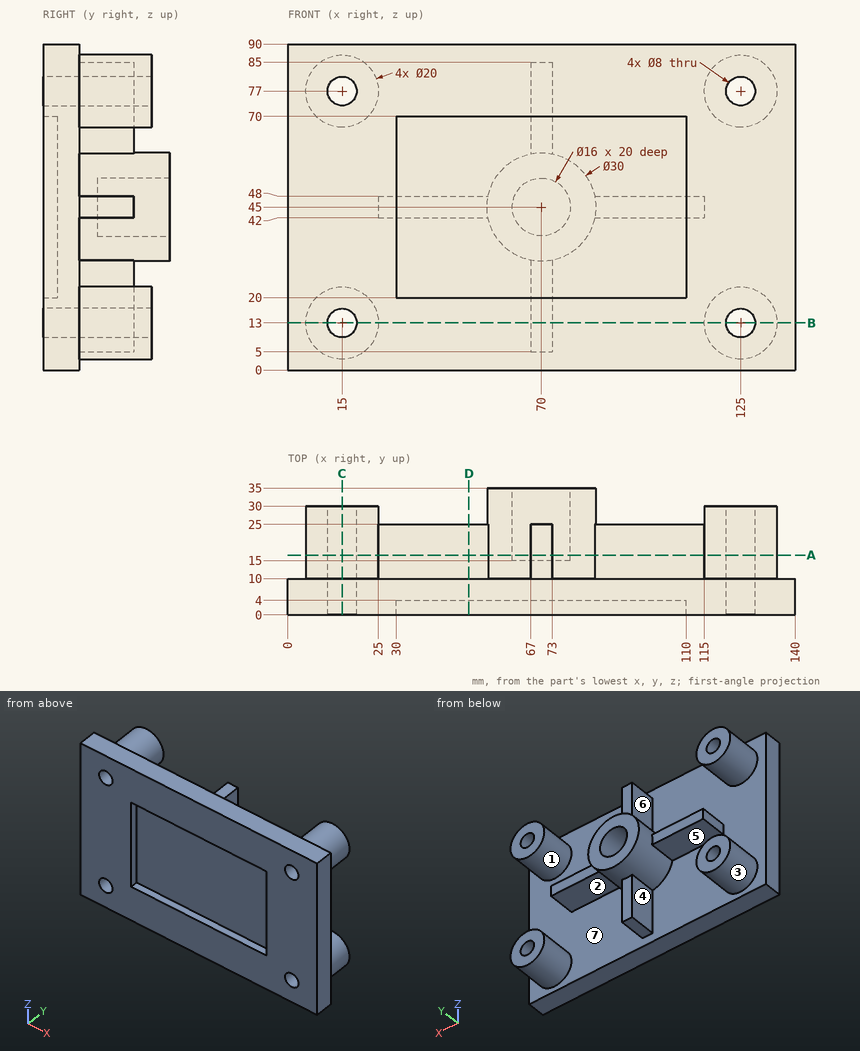
Input: dimensioned drawing with shaded views. Units: mm. Origin: part minimum x, y, z. A direction names the side the tool comes from. Give positions to 0.01 mm unless a question says otherwise; leave off trailing zeros. Write each loop counter-clockwise with the first axis right and the second up, starting at its lowest first coordinate (ties: lowest second). Pieces come first, ordered by that corner, then holes.
1. Reachability of the marked faces 5, 6 and 7 from +Z, -Z, +X, -X, +Y, -Y: full face, straight path, thin tool, end or side. Return the list, or none.
2. Pin query (flat end, axial travel): P1, Ø12, axis at x = 84, z = 33.5, coming from the -Y side; P2, Ø5, axis at y = 18, z = 10.5, coming from the +X side; P3, Ø6.5, axis at x = 40.5, z = 44.5, coming from the +Y side. Return the tip coordinate at first contact, or that it passes through.
3. Line query: probe 1 along X at (y, z) = (10.5, 77); probe 2 along X at (y, z) = (3.5, 31); probe 3 along Z at (x, y) = (17, 23.5). Output: solid intervals per line, ascending.
4. Section query A-A, the plane y = 16.5. Count the separate pieces of the cut face and the enclosed holes in it, then the cut area to 3 significant figures.
5. Section query B-B, the plane z = 13. Return loops of the section in (x, y), then the cut area to 3 significant figures.
6. Draft query along Z for the marked faces 1, 2, 3 and 4. Return one class per face: released by +Z, released by -Z, zero draft, split by the parting line, or undercut.
7. Section query D-D, the plane x = 50. Return loops of the section in (y, z), then the cut area to 3 significant figures.
8. Section query C-C, the plane x = 15. Return loops of the section in (y, z).
Computed:
1. face 5: -Z, -X, +Y
1. face 6: +Z, +Y
1. face 7: +Y
2. P1: stops at y = 4
2. P2: stops at x = 135
2. P3: stops at y = 25
3. probe 1: x = 5 to 11, 19 to 25, 67 to 73, 115 to 121, 129 to 135
3. probe 2: x = 0 to 30, 110 to 140
3. probe 3: z = 3.2 to 9.54, 16.46 to 22.8, 67.2 to 73.54, 80.46 to 86.8
4. separate pieces: 5
4. enclosed holes: 5
4. area: 2,220 mm2
5. outline: (0, 0) - (11, 0) - (11, 30) - (5, 30) - (5, 10) - (0, 10) - close; (19, 0) - (121, 0) - (121, 30) - (115, 30) - (115, 10) - (73, 10) - (73, 25) - (67, 25) - (67, 10) - (25, 10) - (25, 30) - (19, 30) - close; (129, 0) - (140, 0) - (140, 10) - (135, 10) - (135, 30) - (129, 30) - close
5. area: 1,810 mm2
6. face 1: undercut
6. face 2: released by -Z
6. face 3: undercut
6. face 4: zero draft
7. outline: (0, 0) - (10, 0) - (10, 42) - (25, 42) - (25, 48) - (10, 48) - (10, 90) - (0, 90) - (0, 70) - (4, 70) - (4, 20) - (0, 20) - close
7. area: 790 mm2
8. outline: (0, 0) - (10, 0) - (10, 3) - (30, 3) - (30, 9) - (0, 9) - close; (0, 17) - (30, 17) - (30, 23) - (10, 23) - (10, 67) - (30, 67) - (30, 73) - (0, 73) - close; (0, 81) - (30, 81) - (30, 87) - (10, 87) - (10, 90) - (0, 90) - close
